Source: CAD feature listing. Evaluate the final solid. Frame: model axes, mm. Face numbers are marked on the shaded views. A direction names the side the tool comes from. Coordinates: 2 decimals unless noted, no trailing zeros. Write each loop counter-clockwise with the first axis right and the second up, starting at its lowest first coordinate (ties: lowest second). Pieces come first, ordered by that corner, then holes. Notation, with made-up numbers: (67.5, -18) - (124.5, -18) arc R19 ccw to (124.5, 17) - close; hole circle Ø8 at (79.5, 88). An arc over 180 degrees is marked (long way). One line per item, written item: value.
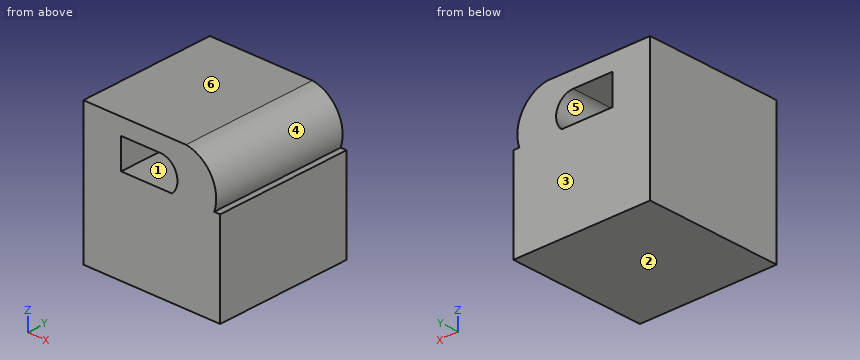
from build123d import *

# Parameters (mm, degrees)
F1_DEPTH = 38.1
F3_DEPTH = 38.1
F5_DEPTH = 25.4
F6_DEPTH = 25.4


with BuildPart() as f1:
    # F0 (on Front) → F1 (new body)
    with BuildSketch(Plane.XZ):
        Polygon((0, 38.099186), (0, 0), (37.85099, 0), (38.1, 38.099186), align=None)
    extrude(amount=F1_DEPTH)

    # F2 (on Front) → F3 (cut)
    with BuildSketch(Plane.XZ):
        with BuildLine():
            Line((10.514395, 33.617546), (10.514395, 24.092546))
            Line((10.514395, 24.092546), (21.440399, 24.092546))
            ThreePointArc((21.440399, 24.092546), (26.202899, 28.855046), (21.440399, 33.617546))
            Line((21.440399, 33.617546), (10.514395, 33.617546))
        make_face()
        with BuildLine():
            Line((10.513219, 14.010213), (10.513219, 4.485213))
            Line((10.513219, 4.485213), (21.435219, 4.485213))
            ThreePointArc((21.435219, 4.485213), (26.197719, 9.247713), (21.435219, 14.010213))
            Line((21.435219, 14.010213), (10.513219, 14.010213))
        make_face()
        with BuildLine():
            Line((38.1, 38.1), (28.575, 38.1))
            ThreePointArc((28.575, 38.1), (36.984506, 28.0415), (27.442695, 19.05))
            ThreePointArc((27.442695, 19.05), (36.984506, 10.0585), (28.575, 0))
            Line((28.575, 0), (38.1, 0))
            Line((38.1, 0), (38.1, 38.1))
        make_face()
    extrude(amount=F3_DEPTH, mode=Mode.SUBTRACT)

    # F4 (on Top) → F5 (join)
    with BuildSketch(Plane.XY):
        Polygon((38.1, 0), (0, 0), (0, -38.1), (38.1, -38.1), (38.1, -30.48), (7.62, -30.48), (7.62, -9.450001), (7.62, -7.62), (38.1, -7.62), align=None)
        Polygon((38.1, -30.48), (38.1, -7.62), (7.62, -7.62), (7.62, -9.450001), (7.62, -30.48), align=None)
    extrude(amount=F5_DEPTH)

    # F4 (on Top) → F6 (join)
    with BuildSketch(Plane.XY):
        Polygon((38.1, 0), (0, 0), (0, -38.1), (38.1, -38.1), (38.1, -30.48), (7.62, -30.48), (7.62, -9.450001), (7.62, -7.62), (38.1, -7.62), align=None)
        Polygon((38.1, -30.48), (38.1, -7.62), (7.62, -7.62), (7.62, -9.450001), (7.62, -30.48), align=None)
    extrude(amount=F6_DEPTH)


solid = f1.part
1) Material intervals for line 1 (Z direction, x = 17.5, y = -26); line 2 (X direction, y = -11, z = 30); line 3 (X direction, y = -17, z = 32), sorted ascending.
Values found:
line 1: 0 to 25.4, 33.62 to 38.1
line 2: 0 to 10.51, 26.06 to 36.9
line 3: 0 to 10.51, 25.02 to 36.38
2) Section query B-B on y = -19.5. Output: boundary loops of the cut face in (x, z) (1 decimal), then the cut area to 3 significant figures.
Values found:
outline: (0, 0) - (38.1, 0) - (38.1, 25.4) - (36.4, 25.4) arc R9.6 ccw to (28.6, 38.1) - (0, 38.1) - close; hole (10.5, 25.4) - (24.7, 25.4) arc R4.8 ccw to (21.4, 33.6) - (10.5, 33.6) - close
area: 1,300 mm2
3) Section query C-C on x = 32. Output: boundary loops of the cut face in (y, z), then the cut area to 3 significant figures.
Values found:
outline: (-38.1, 0) - (0, 0) - (0, 37.01) - (-38.1, 37.01) - close
area: 1,410 mm2
4) Contact query for flat-ended pins moving along their axis: P1, Ø2, axis at x = 32.5, y = -31.5, coming from the +Z side; P2, Ø4, axis at y = -14.5, z = 28, coming from the +X side; P3, Ø0.8, axis at x = 37.5, y = -22.5, coming from the +Z side. Output: stop coordinate, or through.
Values found:
P1: z = 37.26
P2: x = 37
P3: z = 25.4
5) Section query A-A on x = 19. Output: boundary loops of the cut face in (y, z), then the cut area to 3 significant figures.
Values found:
outline: (-38.1, 0) - (0, 0) - (0, 25.4) - (-38.1, 25.4) - close; (-38.1, 33.62) - (0, 33.62) - (0, 38.1) - (-38.1, 38.1) - close
area: 1,140 mm2
6) Reachability of the marked faces 5 and 6 from +Z, -Z, +X, -X, +Y, -Y: full face, straight path, thin tool, end or side. Return the list, or none.
Values found:
face 5: +Y, -Y
face 6: +Z, +X, -X, +Y, -Y
7) Draft query along Z for the marked faces 1, 2, 3 and 4. Return one class per face: released by +Z, released by -Z, zero draft, split by the parting line, or undercut.
Values found:
face 1: undercut
face 2: released by -Z
face 3: zero draft
face 4: undercut
